Here's how the part is built. I have some questions about the finished solid (model axes, mm). Face numbers are marked on the shaded views. A direction names the side the tool comes from. Round coordinates to 2 decimals unless told otherwise and drop trailing zeros. Order: outer loops, then holes, each group sorted by start corner. A loop starts at its lowest first (then second) coordinate and runs counter-clockwise, first axis right, second up. Notation, with made-up numbers: M -19,80.25 L 23,80.25 A28 cw 23,106.25 Z; hole C 86,86 d11. An arc over 180 degrees is marked long. Use one line per item in the form item = value. Start each with the question number.
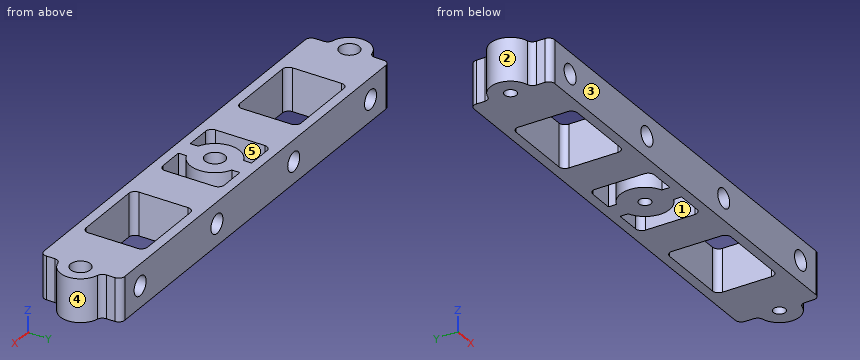
```python
from build123d import *

# Parameters (mm, degrees)
SKETCH1_W           = 195.2625
SKETCH1_H           = 33.3375
SKETCH1_R           = 2.4892
BOSS_EXTRUDE1_DEPTH = 17.78
SKETCH2_R           = 3.96875
CUT_EXTRUDE1_DEPTH  = 33.3375
SKETCH3_R           = 4.064
CUT_EXTRUDE2_DEPTH  = 4.826
CUT_EXTRUDE3_DEPTH  = 17.78
FILLET1_R           = 2.54


with BuildPart() as part:
    # Sketch1 → Boss-Extrude1 (new body)
    with BuildSketch(Plane.XY):
        with Locations((-88.9, 0)):
            Rectangle(SKETCH1_W, SKETCH1_H)
        Circle(SKETCH1_R, mode=Mode.SUBTRACT)
        with Locations((-177.8, 0)):
            Circle(SKETCH1_R, mode=Mode.SUBTRACT)
        with Locations((-88.9, 0)):
            Circle(SKETCH1_R, mode=Mode.SUBTRACT)
    extrude(amount=-BOSS_EXTRUDE1_DEPTH)

    # Sketch2 → Cut-Extrude1 (cut)
    with BuildSketch(Plane(origin=(0, 16.66875, 0), x_dir=(1, 0, 0), z_dir=(0, 1, 0))):
        with Locations(Location((-12.7, 8.89, 0), (0, 0, 270))):
            Circle(SKETCH2_R)
        with Locations(Location((-63.5, 8.89, 0), (0, 0, 270))):
            Circle(SKETCH2_R)
        with Locations(Location((-114.3, 8.89, 0), (0, 0, 270))):
            Circle(SKETCH2_R)
        with Locations(Location((-165.1, 8.89, 0), (0, 0, 270))):
            Circle(SKETCH2_R)
    extrude(amount=-CUT_EXTRUDE1_DEPTH, mode=Mode.SUBTRACT)

    # Sketch3 → Cut-Extrude2 (cut)
    with BuildSketch(Plane.XY):
        Circle(SKETCH3_R)
        with Locations((-88.9, 0)):
            Circle(SKETCH3_R)
        with Locations((-177.8, 0)):
            Circle(SKETCH3_R)
    extrude(amount=-CUT_EXTRUDE2_DEPTH, mode=Mode.SUBTRACT)

    # Sketch5 → Cut-Extrude3 (cut)
    with BuildSketch(Plane.XY):
        with BuildLine():
            Line((0, -16.66875), (8.73125, -16.66875))
            Line((8.73125, -16.66875), (8.73125, 16.66875))
            Line((8.73125, 16.66875), (0, 16.66875))
            Line((0, 16.66875), (0, 10.622546022))
            ThreePointArc((0, 10.622546022), (0.546012526, 9.049137635), (1.949302326, 8.152186482))
            ThreePointArc((1.949302326, 8.152186482), (8.382, 0), (1.949302326, -8.152186482))
            ThreePointArc((1.949302326, -8.152186482), (0.546012526, -9.049137635), (0, -10.622546022))
            Line((0, -10.622546022), (0, -16.66875))
        make_face()
        with BuildLine():
            Line((-23.97125, -12.7), (-52.22875, -12.7))
            ThreePointArc((-52.22875, -12.7), (-54.024801224, -11.956051224), (-54.76875, -10.16))
            Line((-54.76875, -10.16), (-54.76875, 10.16))
            ThreePointArc((-54.76875, 10.16), (-54.024801224, 11.956051224), (-52.22875, 12.7))
            Line((-52.22875, 12.7), (-23.97125, 12.7))
            ThreePointArc((-23.97125, 12.7), (-22.175198776, 11.956051224), (-21.43125, 10.16))
            Line((-21.43125, 10.16), (-21.43125, -10.16))
            ThreePointArc((-21.43125, -10.16), (-22.175198776, -11.956051224), (-23.97125, -12.7))
        make_face()
        with BuildLine():
            Line((-85.011936327, -9.38661605), (-85.011936327, -12.7))
            Line((-85.011936327, -12.7), (-74.77125, -12.7))
            ThreePointArc((-74.77125, -12.7), (-72.975198776, -11.956051224), (-72.23125, -10.16))
            Line((-72.23125, -10.16), (-72.23125, 10.16))
            ThreePointArc((-72.23125, 10.16), (-72.975198776, 11.956051224), (-74.77125, 12.7))
            Line((-74.77125, 12.7), (-85.011936327, 12.7))
            Line((-85.011936327, 12.7), (-85.011936327, 9.38661605))
            ThreePointArc((-85.011936327, 9.38661605), (-78.74, 0), (-85.011936327, -9.38661605))
        make_face()
        with BuildLine():
            Line((-103.02875, 12.7), (-92.788063673, 12.7))
            Line((-92.788063673, 12.7), (-92.788063673, 9.38661605))
            ThreePointArc((-92.788063673, 9.38661605), (-99.06, 0), (-92.788063673, -9.38661605))
            Line((-92.788063673, -9.38661605), (-92.788063673, -12.7))
            Line((-92.788063673, -12.7), (-103.02875, -12.7))
            ThreePointArc((-103.02875, -12.7), (-104.824801224, -11.956051224), (-105.56875, -10.16))
            Line((-105.56875, -10.16), (-105.56875, 10.16))
            ThreePointArc((-105.56875, 10.16), (-104.824801224, 11.956051224), (-103.02875, 12.7))
        make_face()
        with BuildLine():
            Line((-153.82875, 12.7), (-125.57125, 12.7))
            ThreePointArc((-125.57125, 12.7), (-123.775198776, 11.956051224), (-123.03125, 10.16))
            Line((-123.03125, 10.16), (-123.03125, -10.16))
            ThreePointArc((-123.03125, -10.16), (-123.775198776, -11.956051224), (-125.57125, -12.7))
            Line((-125.57125, -12.7), (-153.82875, -12.7))
            ThreePointArc((-153.82875, -12.7), (-155.624801224, -11.956051224), (-156.36875, -10.16))
            Line((-156.36875, -10.16), (-156.36875, 10.16))
            ThreePointArc((-156.36875, 10.16), (-155.624801224, 11.956051224), (-153.82875, 12.7))
        make_face()
        with BuildLine():
            Line((-186.53125, -16.66875), (-186.53125, 16.66875))
            Line((-186.53125, 16.66875), (-177.8, 16.66875))
            Line((-177.8, 16.66875), (-177.8, 10.622546022))
            ThreePointArc((-177.8, 10.622546022), (-178.346012526, 9.049137635), (-179.749302326, 8.152186482))
            ThreePointArc((-179.749302326, 8.152186482), (-186.182, 0), (-179.749302326, -8.152186482))
            ThreePointArc((-179.749302326, -8.152186482), (-178.346012526, -9.049137635), (-177.8, -10.622546022))
            Line((-177.8, -10.622546022), (-177.8, -16.66875))
            Line((-177.8, -16.66875), (-186.53125, -16.66875))
        make_face()
    extrude(amount=-CUT_EXTRUDE3_DEPTH, mode=Mode.SUBTRACT)

    # Fillet1
    fillet1_edges = [part.edges().sort_by_distance(p)[0] for p in [
        (0, 16.66875, -8.89),
        (0, -16.66875, -8.89),
        (-177.8, -16.66875, -8.89),
        (-177.8, 16.66875, -8.89),
    ]]
    fillet(fillet1_edges, radius=FILLET1_R)


solid = part.part
```
1) If I drill on line 1 (X direction, y = -14, z = -9); line 2 (X direction, y = -10.5, z = -13.75); line 3 (Z direction, x = -165.5, y = 15.5), over which ranges is the centre line in solid material (lowest first)?
2) If we section it at D-D on x = -12.7: Write out the boundary of the cut face in (y, z), then the cut area to 3 significant figures.
3) If we mould it in two halves opening along X, with no side actions, what happens to the marked faces 1, 2 and 3? For each: +X half, -X half, draft (parallel to the pull), parting line (faces both ways), or undercut.
4) Will these pins go through, and if not, where does the flat tip stop? pin 1 Ø3 at (y, z) = (12, -5.5) entering from +X; pin 2 Ø1.7 at (y, z) = (11, -10) entering from -X; pin 3 Ø2 at (y, z) = (-2, -11.5) entering from -X.
5) If we section it at B-B on y = 0: Give the number of separate pieces and of enclosed holes in the cut face, then the cut area to 3 significant figures.
6) If we section it at A-A on x = -88.9: Write out the boundary of the cut face in (y, z), then the cut area to 3 significant figures.
7) On a 3-axis mill with a long thin cutter (end or side, diameter ignored), from which of +Z, -Z, +X, -X, +Y, -Y can I reach the whole of each face in a straight line? I mean the marked faces 4 and 5. Say none if no direction works.
Completed:
q1.line_1 = -177.8 to -169.07, -161.13 to -118.27, -110.33 to -67.47, -59.53 to -16.67, -8.73 to 0
q1.line_2 = -177.8 to -156.35, -123.05 to -105.55, -92.79 to -85.01, -72.25 to -54.75, -21.45 to 0
q1.line_3 = -17.78 to -12.84, -4.94 to 0
q2.outline = M -16.67,-17.78 L 16.67,-17.78 L 16.67,-12.86 L -16.67,-12.86 Z; M -16.67,-4.92 L 16.67,-4.92 L 16.67,0 L -16.67,0 Z
q2.area = 328 mm²
q3.face_1 = undercut
q3.face_2 = -X half
q3.face_3 = draft
q4.pin_1 = 0
q4.pin_2 = -177.84
q4.pin_3 = -186.12
q5.separate_pieces = 8
q5.enclosed_holes = 4
q5.area = 1,530 mm²
q6.outline = M -16.67,-17.78 L -2.49,-17.78 L -2.49,-4.83 L -4.06,-4.83 L -4.06,0 L -16.67,0 Z; M 2.49,-17.78 L 16.67,-17.78 L 16.67,0 L 4.06,0 L 4.06,-4.83 L 2.49,-4.83 Z
q6.area = 489 mm²
q7.face_4 = +Z, -Z, +X
q7.face_5 = +Z, -Z
